from build123d import *

# Parameters (mm, degrees)
PAD_DEPTH       = 4
SKETCH_R        = 6
PAD001_DEPTH    = 8
SKETCH002_R     = 3.55
POCKET_DEPTH    = 20
SKETCH003_R     = 1.1
POCKET001_DEPTH = 3.5
FILLET_R        = 0.2
CHAMFER_SIZE    = 0.6


with BuildPart() as part:
    # Sketch001 → Pad (new body)
    with BuildSketch(Plane.XY):
        Polygon((-5, 28), (5, 28), (5, 24), (24, 5), (28, 5), (28, -5), (24, -5), (5, -24), (5, -28), (-5, -28), (-5, -24), (-24, -5), (-28, -5), (-28, 5), (-24, 5), (-5, 24), align=None)
    extrude(amount=PAD_DEPTH)

    # Sketch (on Face18 of Pad) → Pad001 (join)
    with BuildSketch(Plane.XY.offset(4)):
        Circle(SKETCH_R)
    extrude(amount=PAD001_DEPTH)

    # Sketch002 (on Face20 of Pad001) → Pocket (cut)
    with BuildSketch(Plane.XY.offset(12)):
        Circle(SKETCH002_R)
    extrude(amount=-POCKET_DEPTH, mode=Mode.SUBTRACT)

    # Sketch003 (on Face4 of Pocket) → Pocket001 (cut)
    with BuildSketch(Plane(origin=(0, 0, 0), x_dir=(1, 0, 0), z_dir=(0, 0, -1))):
        with Locations((0, 24)):
            Circle(SKETCH003_R)
        with Locations((24, 0)):
            Circle(SKETCH003_R)
        with Locations((-24, 0)):
            Circle(SKETCH003_R)
        with Locations((0, -24)):
            Circle(SKETCH003_R)
    extrude(amount=-POCKET001_DEPTH, mode=Mode.SUBTRACT)

    # Fillet
    fillet_edges = [part.edges().sort_by_distance(p)[0] for p in [
        (28, 0, 4),
        (28, 0, 0),
        (28, 5, 2),
        (26, 5, 4),
        (14.5, 14.5, 4),
        (26, 5, 0),
        (14.5, 14.5, 0),
        (5, 26, 4),
        (5, 26, 0),
        (5, 28, 2),
        (0, 28, 4),
        (0, 28, 0),
        (-5, 28, 2),
        (-5, 26, 4),
        (-14.5, 14.5, 4),
        (-14.5, 14.5, 0),
        (-26, 5, 0),
        (-26, 5, 4),
        (-28, 5, 2),
        (-28, 0, 4),
        (-26, -5, 4),
        (-14.5, -14.5, 4),
        (-5, -26, 4),
        (0, -28, 4),
        (5, -26, 4),
        (14.5, -14.5, 4),
        (26, -5, 4),
        (28, -5, 2),
        (-28, 0, 0),
        (-28, -5, 2),
        (-26, -5, 0),
        (-14.5, -14.5, 0),
        (-5, -26, 0),
        (-5, -28, 2),
        (0, -28, 0),
        (5, -28, 2),
        (14.5, -14.5, 0),
        (5, -26, 0),
        (26, -5, 0),
        (-5, 26, 0),
    ]]
    fillet(fillet_edges, radius=FILLET_R)

    # Chamfer
    chamfer_edges = [part.edges().sort_by_distance(p)[0] for p in [
        (6, 0, 8),
        (-6, 0, 4),
        (-6, 0, 12),
    ]]
    chamfer(chamfer_edges, length=CHAMFER_SIZE)


solid = part.part
The model under review builds one solid part; all positions refer to its coordinate system, in mm. A direction names the side the tool comes from. Round coordinates to 2 decimals unless told otherwise and drop trailing zeros. Write each loop counter-clockwise with the first axis right and the second up, starting at its lowest first coordinate (ties: lowest second). Pieces come first, ordered by that corner, then holes. Notation, with made-up numbers: (25.5, -39.5) - (50.5, -39.5) arc R18 cw to (50.5, -26.5) - close; hole circle Ø8 at (29, 34.5). An arc over 180 degrees is marked (long way). One line per item, written item: value. Start each with the question number.
1. Clearance check with flat-ended pins moving along their axes: P1, Ø2, axis at x = 0, y = 24, coming from the -Z side; P2, Ø1.1, axis at x = 26.5, z = 2, coming from the -Y side; P3, Ø4, axis at x = 27, z = 2.5, coming from the +Y side; P4, Ø1.8, axis at x = 0.5, y = -23.5, coming from the -Z side. State where each tip first meets the part, or that it passes through.
2. Consider section C-C on z = 5.5. Write out the cut boundary in (x, y), and give its area (3 significant figures).
3. The part is to be moulded in two halves that separate along X. For faces 1 (the face through (14.324, -14.591, 0.057)), 2 (the face through (-24, 0, 3.5)), 3 (the face through (-0.238, -22.926, 1.726)), 4 (the face through (-6, 0, 8)), say which applies: released by +X, released by -X, zero draft, split by the parting line, or undercut.
4. Consider section A-A on x = 0. Write out the cut boundary in (y, z).
5. To check wall thickness, follow L1, parallel to X at y = -0.5, z = 1.75; L2, parallel to X at y = -24, z = 1.6. State the ranges of each line that lie inside material, in increasing order. Write a range as from..to.
6. Machinability: for faces 5 (the face through (26, 5, 2)), 6 (the face through (26, -5, 2)), 7 (the face through (-25.1, 0, 1.7)), which of the approach directions +Z, -Z, +X, -X, +Y, -Y give a long, thin tool a straight path to every point of the face, cutting with its end or side? Answer none if there is none.
Checks:
1. P1: stops at z = 3.5
1. P2: stops at y = -5
1. P3: stops at y = 5
1. P4: stops at z = 0
2. outline: circle Ø12 at (0, 0); hole circle Ø7.1 at (0, 0)
2. area: 73.5 mm^2
3. face 1: released by +X
3. face 2: undercut
3. face 3: undercut
3. face 4: split by the parting line
4. outline: (-28, 0.2) arc R0.2 ccw to (-27.8, 0) - (-25.1, 0) - (-25.1, 3.5) - (-22.9, 3.5) - (-22.9, 0) - (-3.55, 0) - (-3.55, 12) - (-5.4, 12) - (-6, 11.4) - (-6, 4.6) - (-6.6, 4) - (-27.8, 4) arc R0.2 ccw to (-28, 3.8) - close; (3.55, 0) - (22.9, 0) - (22.9, 3.5) - (25.1, 3.5) - (25.1, 0) - (27.8, 0) arc R0.2 ccw to (28, 0.2) - (28, 3.8) arc R0.2 ccw to (27.8, 4) - (6.6, 4) - (6, 4.6) - (6, 11.4) - (5.4, 12) - (3.55, 12) - close
5. L1: x = -28..-24.98, -23.02..-3.51, 3.51..23.02, 24.98..28
5. L2: x = -5..-1.1, 1.1..5
6. face 5: +Z, -Z, +X, +Y
6. face 6: +Z, -Z, +X, -Y
6. face 7: -Z
